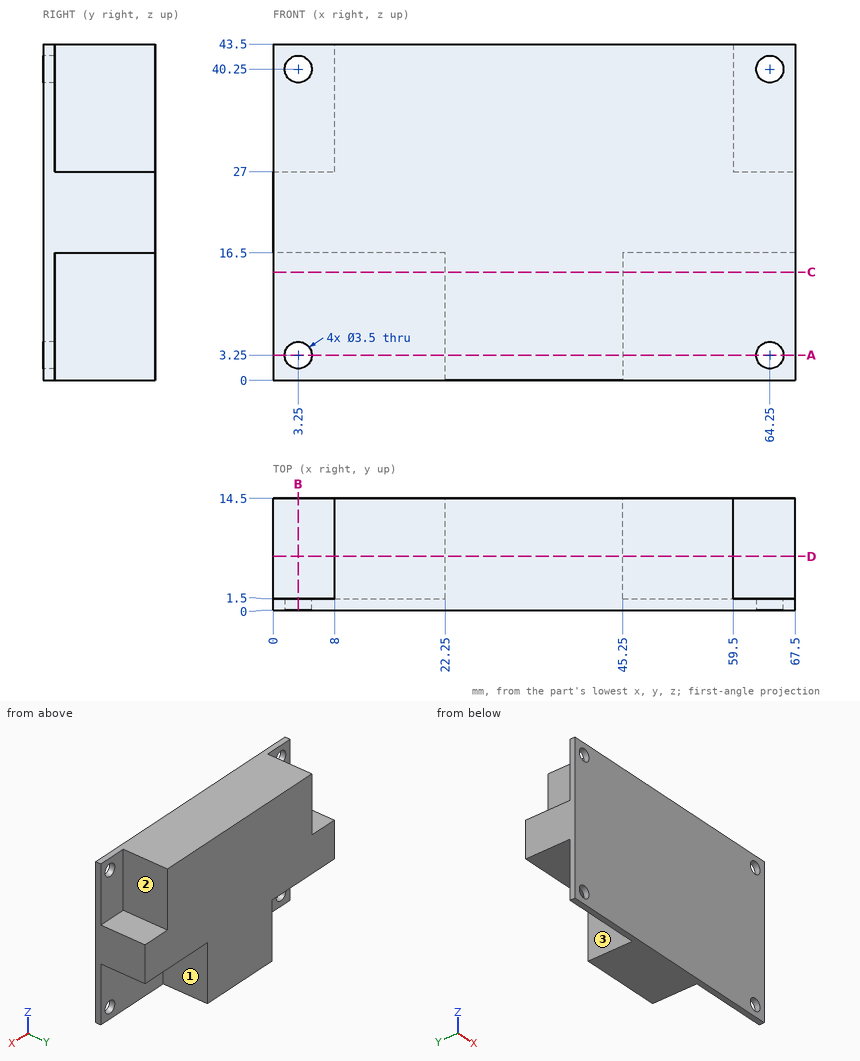
Study the drawing (mm; zero at the part's minimum x, y, z) and answer. A direction names the side the tool comes from. Coordinates: 2 decimals unless noted, no trailing zeros. Write each loop counter-clockwise with the first axis right and the second up, starting at its lowest first coordinate (ties: lowest second). Pieces come first, ordered by that corner, then holes.
Q1. Section B-B, the plane x = 3.25 is taken. Write down the section's boundary in (y, z).
Returned:
outline: (0, 0) - (1.5, 0) - (1.5, 1.5) - (0, 1.5) - close; (0, 5) - (1.5, 5) - (1.5, 16.5) - (14.5, 16.5) - (14.5, 27) - (1.5, 27) - (1.5, 38.5) - (0, 38.5) - close; (0, 42) - (1.5, 42) - (1.5, 43.5) - (0, 43.5) - close
Q2. Which of the six approach directions +Z, -Z, +X, -X, +Y, -Y give full straight-line access (tool end or side, diameter ignored) to the marked faces 1, 2 and 3?
Returned:
face 1: -Z, +X, +Y
face 2: +Z, +X, +Y
face 3: -Z, -X, +Y
Q3. Section C-C, the plane z = 14 is taken. Write down the section's boundary in (x, y), then the cut area to 3 significant figures.
Returned:
outline: (0, 0) - (67.5, 0) - (67.5, 1.5) - (45.25, 1.5) - (45.25, 14.5) - (22.25, 14.5) - (22.25, 1.5) - (0, 1.5) - close
area: 400 mm2
Q4. Section A-A, the plane z = 3.25 is taken. Write down the section's boundary in (x, y), then the cut area to 3 significant figures.
Returned:
outline: (0, 0) - (1.5, 0) - (1.5, 1.5) - (0, 1.5) - close; (5, 0) - (62.5, 0) - (62.5, 1.5) - (45.25, 1.5) - (45.25, 14.5) - (22.25, 14.5) - (22.25, 1.5) - (5, 1.5) - close; (66, 0) - (67.5, 0) - (67.5, 1.5) - (66, 1.5) - close
area: 390 mm2
Q5. Section D-D, the plane y = 7 is taken. Write down the section's boundary in (x, z), then the cut area to 3 significant figures.
Returned:
outline: (0, 16.5) - (22.25, 16.5) - (22.25, 0) - (45.25, 0) - (45.25, 16.5) - (67.5, 16.5) - (67.5, 27) - (59.5, 27) - (59.5, 43.5) - (8, 43.5) - (8, 27) - (0, 27) - close
area: 1,940 mm2
Q6. Find the intervals of material crossed by line 1 along X through (y, z) = (0.6, 3.25); line 2 along Z through (x, y) = (3.25, 0.3); line 3 along X through (y, z) = (7, 7), in increasing order.
Returned:
line 1: x = 0 to 1.5, 5 to 62.5, 66 to 67.5
line 2: z = 0 to 1.5, 5 to 38.5, 42 to 43.5
line 3: x = 22.25 to 45.25
Q7. Given P1, Ø4, axis at x = 64.25, z = 40.25, coming from the +Y side; P2, Ø2, axis at x = 51, y = 13, coming from the -Z side; P3, Ø6.5, axis at x = 3.5, y = 5, coming from the +Z side; P4, Ø3, axis at x = 3.25, z = 3.25, coming from the +Y side, each flat-ended and moving along its own axis, determine where each tip first touches the part or whether it passes through.
Returned:
P1: stops at y = 1.5
P2: stops at z = 16.5
P3: stops at z = 27
P4: passes through
